Model file for the job. Use its own axes, mm. A direction names the side the tool comes from. Coordinates: 2 decimals unless noted, no trailing zeros. Order: outer loops, then holes, each group sorted by start corner. A loop starts at its lowest first (then second) coordinate and runs counter-clockwise, first axis right, second up. Notation, with made-up numbers: (85.25, -5.5) -> (133.25, -5.5) arc R21 ccw to (133.25, 21.5) -> close; hole circle Ø5 at (28, 68). An arc over 180 degrees is marked (long way). Use CSV: the item, a comma, the result in double quotes. Start each with the question number.
(1) Cut at C-C on y = -76.2. Write the cut outline in (x, z) (3 decimals), plus the area to 3 significant figures.
(2) Probe L1, parallel to X at y = -106.5, z = -8.25; L2, parallel to Y at x = 25.5, z = 0.25; L3, parallel to X at y = -187.5, z = -1.5. List the from-to ranges inside material, lowest first.
(3) Pin check, flat tips, straight feed: pin 1 Ø9.5 at (y, z) = (-271.5, -3.5) entering from -X; pin 2 Ø9.5 at (x, z) = (-495, -2) entering from +Y; pin 3 Ø5 at (y, z) = (-294, -2) entering from -X. Stop position of each tip, or through.
(4) Cut at D-D on x = 375. Write the cut outline in (y, z) (3 decimals), plus the area to 3 significant figures.
(5) Tool access for faces 4 (the cylindrical face through (-192.9, 194.8, 0.1)), 5 (the cylindrical face through (529.729, -358.086, 0.133)): list every direction of +Z, -Z, +X, -X, +Y, -Y with a clear straight run to the whole face (end or side of a thin tool).
(6) Cut at A-A on z = 1. Write the cut outline in (x, y).
(7) Cut at B-B on y = 228.6. Write the cut outline in (x, z) (3 decimals).
(8) Pull direction Y, two halves, no side cores. Call faces 1 (the cylindrical face through (-486.271, -149.914, 0.133)), 2 (the cylindrical face through (756.053, 359.894, 0.133)), 3 (the cylindrical face through (-692.47, -64.76, 0.13)): pulls with the +Y half, pulls with the -Y half, needs draft (parallel to the pull), parting line crosses it, or undercut.
```python
from build123d import *

# Parameters (mm, degrees)
F1_DEPTH = 9.525
F2_R     = 38.1
F3_DEPTH = 19.051
F4_R     = 38.1
F5_DEPTH = 19.051
F6_R     = 38.1
F7_DEPTH = 25.4


with BuildPart() as f1:
    # F0 (on Top) → F1 (new body, symmetric)
    with BuildSketch(Plane.XY):
        with BuildLine():
            Line((703.410854, 381), (-235.882083, 381))
            ThreePointArc((-235.882083, 381), (-289.76362, 358.681537), (-312.082083, 304.8))
            Line((-312.082083, 304.8), (-312.082083, 152.4))
            ThreePointArc((-312.082083, 152.4), (-319.521571, 134.439488), (-337.482083, 127))
            Line((-337.482083, 127), (-720.344188, 127))
            ThreePointArc((-720.344188, 127), (-772.402815, 106.44476), (-796.375417, 55.868749))
            Line((-796.375417, 55.868749), (-820.082083, -299.731251))
            ThreePointArc((-820.082083, -299.731251), (-799.695614, -356.858627), (-744.050854, -381))
            Line((-744.050854, -381), (-584.2, -381))
            ThreePointArc((-584.2, -381), (-530.318463, -358.681537), (-508, -304.8))
            Line((-508, -304.8), (-508, -203.2))
            ThreePointArc((-508, -203.2), (-485.681537, -149.318463), (-431.8, -127))
            Line((-431.8, -127), (431.8, -127))
            ThreePointArc((431.8, -127), (485.681537, -149.318463), (508, -203.2))
            Line((508, -203.2), (508, -304.8))
            ThreePointArc((508, -304.8), (530.318463, -358.681537), (584.2, -381))
            Line((584.2, -381), (744.050854, -381))
            ThreePointArc((744.050854, -381), (799.695614, -356.858627), (820.082083, -299.731251))
            Line((820.082083, -299.731251), (779.442083, 309.868749))
            ThreePointArc((779.442083, 309.868749), (755.469482, 360.44476), (703.410854, 381))
        make_face()
    extrude(amount=F1_DEPTH, both=True)

    # F2 (on face) → F3 (cut, through all)
    with BuildSketch(Plane.XY.offset(9.525)):
        with Locations((-210.482083, 228.6)):
            Circle(F2_R)
    extrude(amount=-F3_DEPTH, mode=Mode.SUBTRACT)

    # F4 (on face) → F5 (cut, through all)
    with BuildSketch(Plane.XY.offset(9.525)):
        with Locations((-728.810854, -76.2)):
            Circle(F4_R)
    extrude(amount=-F5_DEPTH, mode=Mode.SUBTRACT)

    # F6 (on face) → F7 (cut)
    with BuildSketch(Plane.XY.offset(9.525)):
        with Locations((728.810854, -76.2)):
            Circle(F6_R)
    extrude(amount=-F7_DEPTH, mode=Mode.SUBTRACT)


solid = f1.part
```
Outcome:
1,outline,"(-805.18, -9.525) -> (-766.911, -9.525) -> (-766.911, 9.525) -> (-805.18, 9.525) -> close; (-690.711, -9.525) -> (690.711, -9.525) -> (690.711, 9.525) -> (-690.711, 9.525) -> close; (766.911, -9.525) -> (805.18, -9.525) -> (805.18, 9.525) -> (766.911, 9.525) -> close"
1,area,"27,800 mm2"
2,L1,"-807.2 to -751.91, -705.71 to 705.71, 751.91 to 807.2"
2,L2,"-127 to 381"
2,L3,"-812.6 to -506.37, 506.37 to 812.6"
3,pin 1,"x = -818.52"
3,pin 2,"y = 127"
3,pin 3,"x = -819.87"
4,outline,"(-127, -9.525) -> (381, -9.525) -> (381, 9.525) -> (-127, 9.525) -> close"
4,area,"9,680 mm2"
5,face 4,"+Z, -Z"
5,face 5,"+Z, -Z, -Y"
6,outline,"(-820.08, -299.73) arc R76.2 ccw to (-744.05, -381) -> (-584.2, -381) arc R76.2 ccw to (-508, -304.8) -> (-508, -203.2) arc R76.2 cw to (-431.8, -127) -> (431.8, -127) arc R76.2 cw to (508, -203.2) -> (508, -304.8) arc R76.2 ccw to (584.2, -381) -> (744.05, -381) arc R76.2 ccw to (820.08, -299.73) -> (779.44, 309.87) arc R76.2 ccw to (703.41, 381) -> (-235.88, 381) arc R76.2 ccw to (-312.08, 304.8) -> (-312.08, 152.4) arc R25.4 cw to (-337.48, 127) -> (-720.34, 127) arc R76.2 ccw to (-796.38, 55.87) -> close; hole circle Ø76.2 at (-728.81, -76.2); hole circle Ø76.2 at (-210.48, 228.6); hole circle Ø76.2 at (728.81, -76.2)"
7,outline,"(-312.082, -9.525) -> (-248.582, -9.525) -> (-248.582, 9.525) -> (-312.082, 9.525) -> close; (-172.382, -9.525) -> (784.86, -9.525) -> (784.86, 9.525) -> (-172.382, 9.525) -> close"
8,face 1,"pulls with the -Y half"
8,face 2,"pulls with the +Y half"
8,face 3,"undercut"
